Design review of the part built by this model. Coordinates are the model's own, in mm. Face numbers are marked on the shaded views. Give positions to 0.01 mm unless a question says otherwise; leave off trailing zeros. Loops run counter-clockwise (first coordinate to the right, second up) from the corner with the lowest first, then second, coordinate; pieces in that order, holes last.
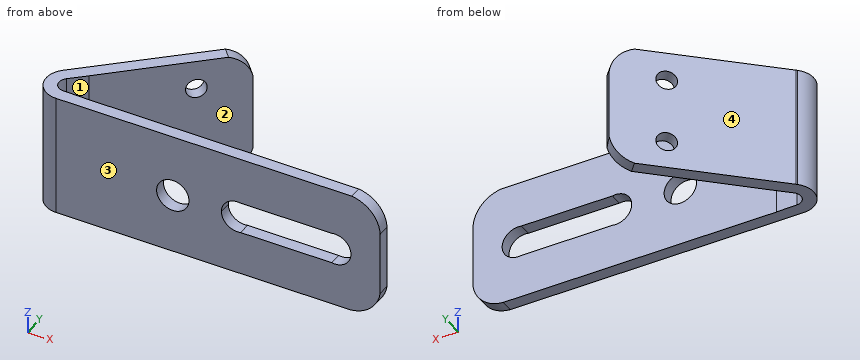
from build123d import *

# Parameters (mm, degrees)
F1_DEPTH  = 483.87
F2_DEPTH  = 483.87
F4_DEPTH  = 50.8
F6_DEPTH  = 50.8
F7_R      = 38.1
F8_DEPTH  = 50.8
F9_R      = 63.5
F10_DEPTH = 76.2
F12_DEPTH = 635


with BuildPart() as f1:
    # F0 (on Top) → F1 (new body)
    with BuildSketch(Plane.XY):
        with BuildLine():
            Line((-634.862884804, -60.9142784472), (-634.862884804, -12.6542784472))
            Line((-634.862884804, -12.6542784472), (-556.1731070353, -12.6542784472))
            ThreePointArc((-556.1731070353, -12.6542784472), (-549.0114244021, 6.7905310299), (-546.5795370493, 27.3690693075))
            ThreePointArc((-546.5795370493, 27.3690693075), (-561.1950321028, 76.0208623801), (-600.2022649901, 108.5638408442))
            ThreePointArc((-600.2022649901, 108.5638408442), (-637.9975803191, 115.5967473616), (-675.1984709822, 105.8992544496))
            Line((-675.1984709822, 105.8992544496), (-694.956899354, 92.0425484629))
            ThreePointArc((-694.956899354, 92.0425484629), (-717.0320418569, -4.9137298277), (-634.862884804, -60.9142784472))
        make_face()
        with BuildLine():
            ThreePointArc((-596.762884804, 27.3690693075), (-654.0657903767, -5.5377448435), (-653.6058463562, 60.5400112937))
            ThreePointArc((-653.6058463562, 60.5400112937), (-615.6599792314, 60.2758834585), (-596.762884804, 27.3690693075))
        make_face(mode=Mode.SUBTRACT)
        with BuildLine():
            Line((-556.1731070353, -12.6542784472), (-634.862884804, -12.6542784472))
            Line((-634.862884804, -12.6542784472), (-634.862884804, -60.9142784472))
            ThreePointArc((-634.862884804, -60.9142784472), (-588.7079589421, -47.8883044805), (-556.1731070353, -12.6542784472))
        make_face()
        with BuildLine():
            Line((635.137115196, -12.6542784472), (-556.1731070353, -12.6542784472))
            ThreePointArc((-556.1731070353, -12.6542784472), (-588.7079589421, -47.8883044805), (-634.862884804, -60.9142784472))
            Line((-634.862884804, -60.9142784472), (635.137115196, -60.9142784472))
            Line((635.137115196, -60.9142784472), (635.137115196, -12.6542784472))
        make_face()
        with BuildLine():
            Line((-692.2264455581, 94.4762327731), (-694.956899354, 92.0425484629))
            Line((-694.956899354, 92.0425484629), (-675.1984709822, 105.8992544496))
            ThreePointArc((-675.1984709822, 105.8992544496), (-684.0452209002, 100.6837834303), (-692.2264455581, 94.4762327731))
        make_face()
        with BuildLine():
            ThreePointArc((-692.2264455581, 94.4762327731), (-693.6042773982, 93.273532638), (-694.956899354, 92.0425484629))
            Line((-694.956899354, 92.0425484629), (-692.2264455581, 94.4762327731))
        make_face()
        with BuildLine():
            ThreePointArc((-675.1984709822, 105.8992544496), (-637.9975803191, 115.5967473616), (-600.2022649901, 108.5638408442))
            Line((-600.2022649901, 108.5638408442), (-173.0680713738, 492.6695353448))
            Line((-173.0680713738, 492.6695353448), (-203.0335409277, 530.4993943773))
            Line((-203.0335409277, 530.4993943773), (-692.2264455581, 94.4762327731))
            ThreePointArc((-692.2264455581, 94.4762327731), (-684.0452209002, 100.6837834303), (-675.1984709822, 105.8992544496))
        make_face()
    extrude(amount=F1_DEPTH)

    # F0 (on Top) → F2 (join)
    with BuildSketch(Plane.XY):
        with BuildLine():
            Line((-634.862884804, -60.9142784472), (-634.862884804, -12.6542784472))
            Line((-634.862884804, -12.6542784472), (-556.1731070353, -12.6542784472))
            ThreePointArc((-556.1731070353, -12.6542784472), (-549.0114244021, 6.7905310299), (-546.5795370493, 27.3690693075))
            ThreePointArc((-546.5795370493, 27.3690693075), (-561.1950321028, 76.0208623801), (-600.2022649901, 108.5638408442))
            ThreePointArc((-600.2022649901, 108.5638408442), (-637.9975803191, 115.5967473616), (-675.1984709822, 105.8992544496))
            Line((-675.1984709822, 105.8992544496), (-694.956899354, 92.0425484629))
            ThreePointArc((-694.956899354, 92.0425484629), (-717.0320418569, -4.9137298277), (-634.862884804, -60.9142784472))
        make_face()
        with BuildLine():
            ThreePointArc((-596.762884804, 27.3690693075), (-654.0657903767, -5.5377448435), (-653.6058463562, 60.5400112937))
            ThreePointArc((-653.6058463562, 60.5400112937), (-615.6599792314, 60.2758834585), (-596.762884804, 27.3690693075))
        make_face(mode=Mode.SUBTRACT)
        with BuildLine():
            Line((-556.1731070353, -12.6542784472), (-634.862884804, -12.6542784472))
            Line((-634.862884804, -12.6542784472), (-634.862884804, -60.9142784472))
            ThreePointArc((-634.862884804, -60.9142784472), (-588.7079589421, -47.8883044805), (-556.1731070353, -12.6542784472))
        make_face()
        with BuildLine():
            Line((635.137115196, -12.6542784472), (-556.1731070353, -12.6542784472))
            ThreePointArc((-556.1731070353, -12.6542784472), (-588.7079589421, -47.8883044805), (-634.862884804, -60.9142784472))
            Line((-634.862884804, -60.9142784472), (635.137115196, -60.9142784472))
            Line((635.137115196, -60.9142784472), (635.137115196, -12.6542784472))
        make_face()
        with BuildLine():
            Line((-692.2264455581, 94.4762327731), (-694.956899354, 92.0425484629))
            Line((-694.956899354, 92.0425484629), (-675.1984709822, 105.8992544496))
            ThreePointArc((-675.1984709822, 105.8992544496), (-684.0452209002, 100.6837834303), (-692.2264455581, 94.4762327731))
        make_face()
        with BuildLine():
            ThreePointArc((-692.2264455581, 94.4762327731), (-693.6042773982, 93.273532638), (-694.956899354, 92.0425484629))
            Line((-694.956899354, 92.0425484629), (-692.2264455581, 94.4762327731))
        make_face()
        with BuildLine():
            ThreePointArc((-675.1984709822, 105.8992544496), (-637.9975803191, 115.5967473616), (-600.2022649901, 108.5638408442))
            Line((-600.2022649901, 108.5638408442), (-173.0680713738, 492.6695353448))
            Line((-173.0680713738, 492.6695353448), (-203.0335409277, 530.4993943773))
            Line((-203.0335409277, 530.4993943773), (-692.2264455581, 94.4762327731))
            ThreePointArc((-692.2264455581, 94.4762327731), (-684.0452209002, 100.6837834303), (-675.1984709822, 105.8992544496))
        make_face()
    extrude(amount=F2_DEPTH)

    # F3 (on face) → F4 (cut)
    with BuildSketch(Plane(origin=(-353.3908608831, 396.4842167311, 0), x_dir=(-0.7465106955, -0.6653734151, 0), z_dir=(-0.6653734151, 0.7465106955, 0))):
        with BuildLine():
            ThreePointArc((-112.7163544297, 0), (-170.8315172722, 36.574359485), (-201.4134839174, 98.0544313788))
            Line((-201.4134839174, 98.0544313788), (-201.4134839174, 0))
            Line((-201.4134839174, 0), (-112.7163544297, 0))
        make_face()
        with BuildLine():
            Line((-201.4134839174, 483.87), (-201.4134839174, 376.6429126263))
            ThreePointArc((-201.4134839174, 376.6429126263), (-173.0583201372, 443.4860309567), (-112.7163544297, 483.87))
            Line((-112.7163544297, 483.87), (-201.4134839174, 483.87))
        make_face()
    extrude(amount=-F4_DEPTH, mode=Mode.SUBTRACT)

    # F5 (on face) → F6 (cut)
    with BuildSketch(Plane.XZ.offset(60.9142784472)):
        with BuildLine():
            Line((635.137115196, 0), (635.137115196, 110.7464699671))
            ThreePointArc((635.137115196, 110.7464699671), (595.8393127678, 33.9689040087), (516.5598988533, 0))
            Line((516.5598988533, 0), (635.137115196, 0))
        make_face()
        with BuildLine():
            ThreePointArc((524.1865515709, 483.87), (602.2885378872, 443.1693633222), (635.137115196, 361.4538013935))
            Line((635.137115196, 361.4538013935), (635.137115196, 483.87))
            Line((635.137115196, 483.87), (524.1865515709, 483.87))
        make_face()
    extrude(amount=-F6_DEPTH, mode=Mode.SUBTRACT)

    # F7 (on face) → F8 (cut)
    with BuildSketch(Plane(origin=(-353.3908608831, 396.4842167311, 0), x_dir=(-0.7465106955, -0.6653734151, 0), z_dir=(-0.6653734151, 0.7465106955, 0))):
        with Locations((0, 369.57)):
            Circle(F7_R)
        with Locations((0, 109.4054887733)):
            Circle(F7_R)
    extrude(amount=-F8_DEPTH, mode=Mode.SUBTRACT)

    # F9 (on face) → F10 (cut)
    with BuildSketch(Plane(origin=(0, -12.6542784472, 0), x_dir=(-1, 0, 0), z_dir=(0, 1, 0))):
        with BuildLine():
            Line((-76.337115196, 173.7487316132), (-76.337115196, 298.4515397475))
            Line((-76.337115196, 298.4515397475), (-88.3601102827, 298.4515397475))
            ThreePointArc((-88.3601102827, 298.4515397475), (-139.837115196, 236.1001356803), (-88.3601102827, 173.7487316132))
            Line((-88.3601102827, 173.7487316132), (-76.337115196, 173.7487316132))
        make_face()
        with BuildLine():
            Line((-88.3601102827, 298.4515397475), (-76.337115196, 298.4515397475))
            Line((-76.337115196, 298.4515397475), (-76.337115196, 173.7487316132))
            Line((-76.337115196, 173.7487316132), (-88.3601102827, 173.7487316132))
            ThreePointArc((-88.3601102827, 173.7487316132), (-35.9094649304, 187.1322370731), (-12.837115196, 236.1001356803))
            ThreePointArc((-12.837115196, 236.1001356803), (-35.9094649304, 285.0680342875), (-88.3601102827, 298.4515397475))
        make_face()
        with BuildLine():
            Line((-457.337115196, 298.4515397475), (-445.3141201093, 298.4515397475))
            ThreePointArc((-445.3141201093, 298.4515397475), (-520.837115196, 236.1001356803), (-445.3141201093, 173.7487316132))
            Line((-445.3141201093, 173.7487316132), (-457.337115196, 173.7487316132))
            Line((-457.337115196, 173.7487316132), (-457.337115196, 298.4515397475))
        make_face()
        with BuildLine():
            ThreePointArc((-393.837115196, 236.1001356803), (-408.3692165888, 276.5277859459), (-445.3141201093, 298.4515397475))
            Line((-445.3141201093, 298.4515397475), (-457.337115196, 298.4515397475))
            Line((-457.337115196, 298.4515397475), (-457.337115196, 173.7487316132))
            Line((-457.337115196, 173.7487316132), (-445.3141201093, 173.7487316132))
            ThreePointArc((-445.3141201093, 173.7487316132), (-408.3692165888, 195.6724854147), (-393.837115196, 236.1001356803))
        make_face()
        with BuildLine():
            ThreePointArc((-88.3601102827, 173.7487316132), (-139.837115196, 236.1001356803), (-88.3601102827, 298.4515397475))
            Line((-88.3601102827, 298.4515397475), (-445.3141201093, 298.4515397475))
            ThreePointArc((-445.3141201093, 298.4515397475), (-408.3692165888, 276.5277859459), (-393.837115196, 236.1001356803))
            ThreePointArc((-393.837115196, 236.1001356803), (-408.3692165888, 195.6724854147), (-445.3141201093, 173.7487316132))
            Line((-445.3141201093, 173.7487316132), (-88.3601102827, 173.7487316132))
        make_face()
        with Locations((177.662884804, 236.1001356803)):
            Circle(F9_R)
    extrude(amount=-F10_DEPTH, mode=Mode.SUBTRACT)

    # F11 (on face) → F12 (cut)
    with BuildSketch(Plane.XY.offset(483.87)):
        Polygon((-518.1578993797, 89.6325483918), (-600.2022649901, 108.5638408442), (-660.0170895818, 55.9850784981), (-635.4890244176, -10.7257853212), (-518.1578993797, -12.6542784472), align=None)
    extrude(amount=-F12_DEPTH, mode=Mode.SUBTRACT)


solid = f1.part
Q1. Take a section at D-D (z = 450). Give the boundary of the cut face in (x, y).
Results:
outline: (-692.23, 94.48) arc R88.28 ccw to (-634.86, -60.91) - (595.61, -60.91) - (595.61, -12.65) - (-556.17, -12.65) arc R88.28 ccw to (-555.86, -12.03) - (-635.49, -10.73) arc R38.1 cw to (-660.02, 55.99) - (-600.2, 108.56) - (-196.36, 471.72) - (-228.51, 507.79) - close
Q2. Wall thickness on line 1 (Y direction, x = -41.5, z = 324); line 2 (Y direction, x = -465, z = 160); line 3 (Y direction, x = -658.5, z = 299): over which ranges is each line inside the solid? List them lowest first.
Results:
line 1: y = -60.91 to -12.65
line 2: y = -60.91 to -12.65, 230.15 to 297.01
line 3: y = -57.69 to -2.51, 57.32 to 124.54
Q3. Take a section at B-B (z = 262). Give the boundary of the cut face in (x, y).
Results:
outline: (-692.23, 94.48) arc R88.28 ccw to (-634.86, -60.91) - (-235.64, -60.91) - (-235.64, -12.65) - (-556.17, -12.65) arc R88.28 ccw to (-555.86, -12.03) - (-635.49, -10.73) arc R38.1 cw to (-660.02, 55.99) - (-600.2, 108.56) - (-173.07, 492.67) - (-203.03, 530.5) - close; (-119.68, -60.91) - (18.36, -60.91) - (18.36, -12.65) - (-119.68, -12.65) - close; (515.32, -60.91) - (635.14, -60.91) - (635.14, -12.65) - (515.32, -12.65) - close
Q4. Take a section at C-C (x = -487). Give the boundary of the cut face in (y, z), plus the area to 3 significant figures.
Results:
outline: (-60.91, 0) - (-12.65, 0) - (-12.65, 483.87) - (-60.91, 483.87) - close; (210.36, 0) - (277.4, 0) - (277.4, 483.87) - (210.36, 483.87) - close
area: 55,800 mm2
Q5. Take a section at A-A (x = 206.5). Give the boundary of the cut face in (y, z), plus the area to 3 significant figures.
Results:
outline: (-60.91, 0) - (-12.65, 0) - (-12.65, 173.75) - (-60.91, 173.75) - close; (-60.91, 298.45) - (-12.65, 298.45) - (-12.65, 483.87) - (-60.91, 483.87) - close
area: 17,300 mm2
Q6. Insertion check: pin 1 (2 mm diameter, centred on x = 291, z = 123, fed in from +Y); pin 2 (2 mm diameter, centred on y = 397, z = 336.5, fed in from +X); pin 3 (3 mm diameter, centred on x = -440.5, z = 191.5, fed in from +Y). Each pin has a flat end and moves straight along its axis. Give the tip position at first contact, or say it passes through.
Results:
pin 1: stops at y = -12.65
pin 2: stops at x = -278.34
pin 3: stops at y = 320.18
Q7. Draft analysis for pull direction Y (two halves, no side actions). For the marked faces 1, 2, 3 and 4, state which applies: pulls with the +Y half, pulls with the -Y half, needs draft (parallel to the pull), parting line crosses it, or undercut.
Results:
face 1: undercut
face 2: undercut
face 3: pulls with the -Y half
face 4: pulls with the +Y half
